```python
from build123d import *

# Parameters (mm, degrees)
SALIENTE_EXTRUIR1_DEPTH = 1.5
CROQUIS2_W              = 30
CROQUIS2_H              = 3.1
CORTAR_EXTRUIR1_DEPTH   = 10
CROQUIS3_R              = 1.5
CORTAR_EXTRUIR2_DEPTH   = 3
CROQUIS6_R              = 1.5
CORTAR_EXTRUIR3_DEPTH   = 3
CROQUIS8_R              = 1.5
CORTAR_EXTRUIR4_DEPTH   = 3


with BuildPart() as part:
    # Croquis1 → Saliente-Extruir1 (new, symmetric)
    with BuildSketch(Plane.XY):
        Polygon((-100, -27), (-100, -45), (-71.428571429, -45), (-71.428571429, -41.9), (-42.857142857, -41.9), (-42.857142857, -45), (-14.285714286, -45), (-14.285714286, -41.9), (14.285714286, -41.9), (14.285714286, -45), (42.857142857, -45), (42.857142857, -41.9), (71.428571429, -41.9), (71.428571429, -45), (100, -45), (100, -27), (96.9, -27), (96.9, -9), (100, -9), (100, 9), (96.9, 9), (96.9, 27), (100, 27), (100, 45), (71.428571429, 45), (71.428571429, 41.9), (42.857142857, 41.9), (42.857142857, 45), (14.285714286, 45), (14.285714286, 41.9), (-14.285714286, 41.9), (-14.285714286, 45), (-42.857142857, 45), (-42.857142857, 41.9), (-71.428571429, 41.9), (-71.428571429, 45), (-100, 45), (-100, 27), (-96.9, 27), (-96.9, 9), (-100, 9), (-100, -9), (-96.9, -9), (-96.9, -27), align=None)
    extrude(amount=SALIENTE_EXTRUIR1_DEPTH, both=True)

    # Croquis2 → Cortar-Extruir1 (cut)
    with BuildSketch(Plane.XY.offset(1.5)):
        with Locations((-60, -25.45)):
            Rectangle(CROQUIS2_W, CROQUIS2_H)
        with Locations((60, -25.45)):
            Rectangle(CROQUIS2_W, CROQUIS2_H)
    extrude(amount=-CORTAR_EXTRUIR1_DEPTH, mode=Mode.SUBTRACT)

    # Croquis3 → Cortar-Extruir2 (cut)
    with BuildSketch(Plane.XY.offset(1.5)):
        with Locations((-82.180986704, 23.889608573)):
            Circle(CROQUIS3_R)
        with Locations((-53.680986704, 23.889608573)):
            Circle(CROQUIS3_R)
        with Locations((-53.680986704, 7.889608573)):
            Circle(CROQUIS3_R)
        with Locations((-82.180986704, 7.889608573)):
            Circle(CROQUIS3_R)
    extrude(amount=-CORTAR_EXTRUIR2_DEPTH, mode=Mode.SUBTRACT)

    # Croquis6 → Cortar-Extruir3 (cut)
    with BuildSketch(Plane.XY.offset(1.5)):
        with Locations((-7.971882846, 34.085861189)):
            Circle(CROQUIS6_R)
        with Locations((-7.971882846, -13.414138811)):
            Circle(CROQUIS6_R)
    extrude(amount=-CORTAR_EXTRUIR3_DEPTH, mode=Mode.SUBTRACT)

    # Croquis8 → Cortar-Extruir4 (cut)
    with BuildSketch(Plane.XY.offset(1.5)):
        with Locations((42.028117154, 19.785861189)):
            Circle(CROQUIS8_R)
        with Locations((42.028117154, -9.414138811)):
            Circle(CROQUIS8_R)
    extrude(amount=-CORTAR_EXTRUIR4_DEPTH, mode=Mode.SUBTRACT)


solid = part.part
```
Here's how the part is built. I have some questions about the finished solid (model axes, mm). Round coordinates to 2 decimals unless told otherwise and drop trailing zeros. Write each loop counter-clockwise with the first axis right and the second up, starting at its lowest first coordinate (ties: lowest second). Pieces come first, ordered by that corner, then holes.
Q1. If we section it at B-B on y = 14: Write out the boundary of the cut face in (x, z).
Q2. Please list where these lines run through material, in increasing order: probe 1 along X at (y, z) = (-26, 1.2); probe 2 along Y at (x, z) = (59.5, 0.6); probe 3 along Y at (x, z) = (-1, 0.7).
Q3. If we section it at C-C on z = -0.95: Give the number of separate pieces and of enclosed holes in the cut face, plus the area to 3 significant figures.
Q4. Will these pins go through, and if not, where does the flat tip stop? P1, Ø1, axis at y = 24.5, z = -1, coming from the -X side; P2, Ø0.9, axis at x = 58, z = 0, coming from the +Y side; P3, Ø1.5, axis at x = -58.5, z = -0.5, coming from the -Y side; P4, Ø1.8, axis at x = -82.18, y = 7.89, coming from the -Z side.
Q5. If we section it at A-A on x = 66.5: Write out the boundary of the cut face in (y, z).
Answer below:
1. outline: (-96.9, -1.5) - (96.9, -1.5) - (96.9, 1.5) - (-96.9, 1.5) - close
2. probe 1: x = -96.9 to -75, -45 to 45, 75 to 96.9
2. probe 2: y = -41.9 to -27, -23.9 to 41.9
2. probe 3: y = -41.9 to 41.9
3. separate pieces: 1
3. enclosed holes: 10
3. area: 17,000 mm2
4. P1: stops at x = -96.9
4. P2: stops at y = 41.9
4. P3: stops at y = -41.9
4. P4: passes through
5. outline: (-41.9, -1.5) - (-27, -1.5) - (-27, 1.5) - (-41.9, 1.5) - close; (-23.9, -1.5) - (41.9, -1.5) - (41.9, 1.5) - (-23.9, 1.5) - close
